Input: part model. Units: mm. Frame: model coordinates. Face numbers are marked on the shaded views. A direction names the side the tool comes from. Give positions to 0.01 mm unless a question says otherwise; leave off trailing zeros. Loops run counter-clockwise (first coordinate to the right, second up) from the corner with the lowest first, then second, coordinate; pieces in that order, holes last. Notation, with made-up numbers: (-14.5, 2.5) -> (-8.5, 2.5) arc R18 cw to (-8.5, 22.5) -> close; hole circle Ø8 at (-1, 60). An arc over 180 degrees is marked (long way). One line per question, with ' | ' between items.
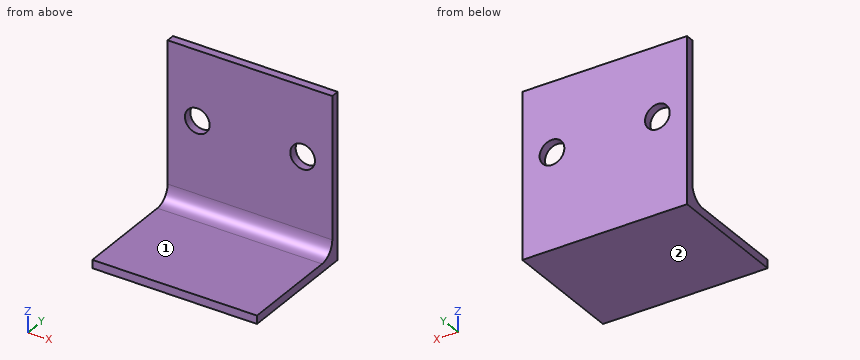
from build123d import *

# Parameters (mm, degrees)
F0_W     = 100
F0_H     = 5
F1_DEPTH = 75
F0_H_2   = 95
F2_DEPTH = 5
F3_R     = 9.5
F4_R     = 7.5
F5_DEPTH = 5.001


with BuildPart() as f1:
    # F0 (on Front) → F1 (new body)
    with BuildSketch(Plane.XZ):
        with Locations((-11.639485, -19.803855)):
            Rectangle(F0_W, F0_H)
    extrude(amount=F1_DEPTH)

    # F0 (on Front) → F2 (join)
    with BuildSketch(Plane.XZ):
        with Locations((-11.639485, 30.196145)):
            Rectangle(F0_W, F0_H_2)
        with Locations((-11.639485, -19.803855)):
            Rectangle(F0_W, F0_H)
    extrude(amount=F2_DEPTH)

    # F3
    f3_edges = [f1.edges().sort_by_distance(p)[0] for p in [
        (-11.639485, -5, -17.303855),
    ]]
    fillet(f3_edges, radius=F3_R)

    # F4 (on face) → F5 (cut, through all)
    with BuildSketch(Plane.XZ.offset(5)):
        with Locations((20.360515, 35.696145)):
            Circle(F4_R)
        with Locations((-43.639485, 35.696145)):
            Circle(F4_R)
    extrude(amount=-F5_DEPTH, mode=Mode.SUBTRACT)


solid = f1.part
1. Reachability of the marked faces 1 and 2 from +Z, -Z, +X, -X, +Y, -Y: full face, straight path, thin tool, end or side. Return the list, or none.
Determined:
face 1: +Z, +X, -X, -Y | face 2: -Z, +X, -X, +Y, -Y
2. Section query D-D (z = -1). Output: boundary loops of the cut face in (x, y), then the cut area to 3 significant figures.
Determined:
outline: (-61.64, -5) -> (38.36, -5) -> (38.36, 0) -> (-61.64, 0) -> close | area: 500 mm2
3. Section query C-C (y = -63). Output: boundary loops of the cut face in (x, z).
Determined:
outline: (-61.64, -22.3) -> (38.36, -22.3) -> (38.36, -17.3) -> (-61.64, -17.3) -> close
4. Section query A-A (x = 22.5). Output: boundary loops of the cut face in (y, z), then the cut area to 3 significant figures.
Determined:
outline: (-75, -22.3) -> (0, -22.3) -> (0, 28.51) -> (-5, 28.51) -> (-5, -7.8) arc R9.5 cw to (-14.5, -17.3) -> (-75, -17.3) -> close; (-5, 42.88) -> (0, 42.88) -> (0, 77.7) -> (-5, 77.7) -> close | area: 797 mm2
5. Pin query (flat end, axial travel): P1, Ø3, axis at x = 14, y = -24.5, coming from the +Z side; P2, Ø12, axis at x = 20.36, z = 35.7, coming from the +Y side; P3, Ø24, axis at x = -43.64, z = 35.7, coming from the -Y side. Return the tip coordinate at first contact, or that it passes through.
Determined:
P1: stops at z = -17.3 | P2: passes through | P3: stops at y = -5
6. Ray query, line 1 along Y through (x, z) = (15.5, -3.5); line 2 along Z through (x, y) = (13.5, -33); line 3 along Y through (x, z) = (-51, -16). Return the intervals inside material, ascending. Write a range as from..to.
Determined:
line 1: y = -5..0 | line 2: z = -22.3..-17.3 | line 3: y = -9.7..0
7. Section query B-B (x = 10). Output: boundary loops of the cut face in (y, z), then the cut area to 3 significant figures.
Determined:
outline: (-75, -22.3) -> (0, -22.3) -> (0, 77.7) -> (-5, 77.7) -> (-5, -7.8) arc R9.5 cw to (-14.5, -17.3) -> (-75, -17.3) -> close | area: 869 mm2
